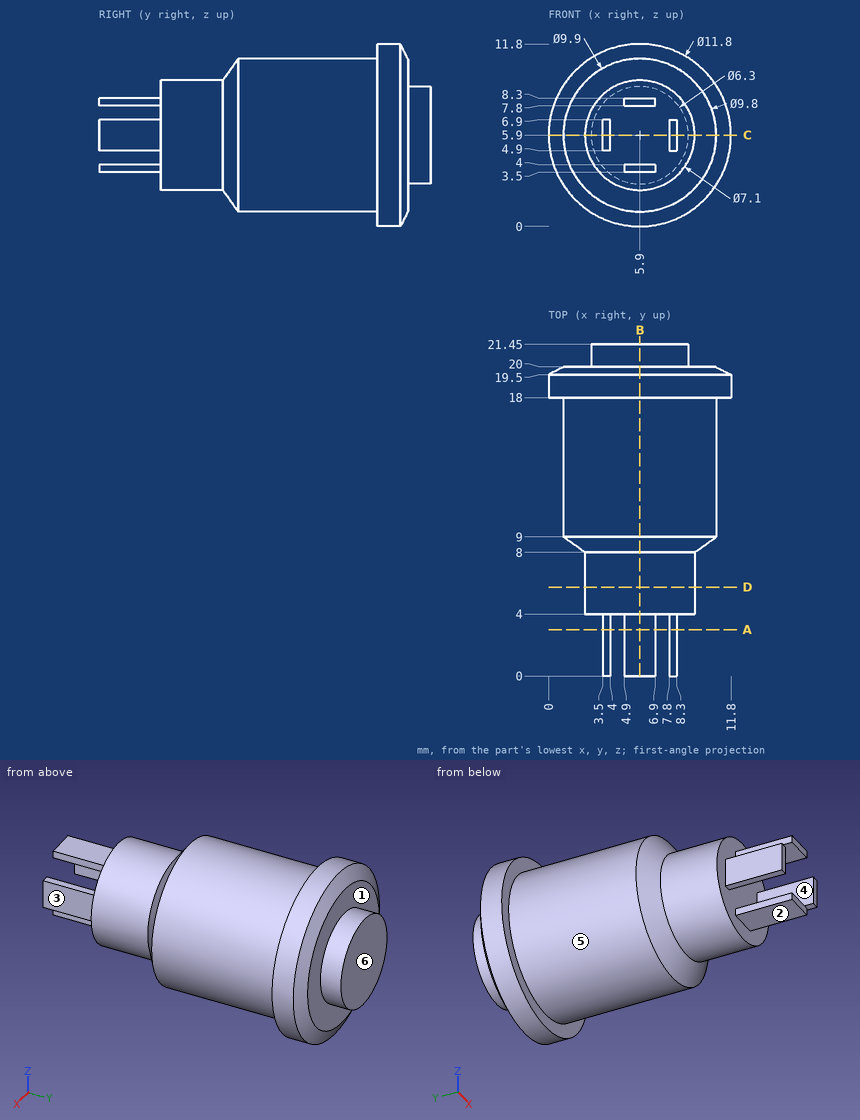
Input: dimensioned drawing with shaded views. Units: mm. Origin: part minimum x, y, z. A direction names the side the tool comes from. Coordinates: 2 decimals unless noted, no trailing zeros. Write each loop counter-clockwise with the first axis right and the second up, starting at its lowest first coordinate (ties: lowest second). Pieces come first, ordered by that corner, then holes. Notation, with made-up numbers: M 74.5,48.25 L 88.5,48.25 A34 cw 88.5,78.25 Z; hole C -12,-29.75 d1. An arc over 180 degrees is marked long. Answer as CSV lines item,"result". Start each with the question number.
Q1. Cut plane D-D on y = 5.75. Return the cut outline in (x, z), then the cut area to 3 significant figures.
Q2. Line query: line 1 (Y direction, x = 4.75, z = 7.5); line 2 (X direction, y = 2.5, z = 8); line 3 (X direction, y = 13.5, z = 4.75). Output: solid intervals per line, ascending. Write a range as from..to.
Q3. Cut plane A-A on y = 3. Return the cut outline in (x, z), then the cut area to 3 significant figures.
Q4. Cut plane C-C on z = 5.9. Return the cut outline in (x, y), then the cut area to 3 significant figures.
Q5. Pin query (flat end, axial travel): P1, Ø6, axis at y = 12.5, z = 1.5, coming from the -X side; P2, Ø0.6, axis at x = 8, y = 1, coming from the -Z side; P3, Ø2, axis at x = 6, y = 2.5, coming from the +Z side. Return the tip coordinate at first contact, or that it passes through.
Q6. Cut plane B-B on x = 5.9. Return the cut outline in (y, z).
Q7. Reachability of the marked faces 1, 2 and 3 from +Z, -Z, +X, -X, +Y, -Y: full face, straight path, thin tool, end or side. Return the list, or none.
Q8. Mould query, pull axis X, two halves, no side actions, for the marked faces 4, 5 and 6. Classes: released by +X, released by -X, zero draft, split by the parting line, or undercut.
Findings below:
1,outline,"C 5.9,5.9 d7.1"
1,area,"39.6 mm2"
2,line 1,"y = 4..21.45"
2,line 2,"x = 4.9..6.9"
2,line 3,"x = 1.09..10.71"
3,outline,"M 3.5,4.9 L 4,4.9 L 4,6.9 L 3.5,6.9 Z; M 4.9,3.5 L 6.9,3.5 L 6.9,4 L 4.9,4 Z; M 4.9,7.8 L 6.9,7.8 L 6.9,8.3 L 4.9,8.3 Z; M 7.8,4.9 L 8.3,4.9 L 8.3,6.9 L 7.8,6.9 Z"
3,area,"4.00 mm2"
4,outline,"M 0,18 L 0.95,18 L 0.95,9 L 2.35,8 L 2.35,4 L 3.5,4 L 3.5,0 L 4,0 L 4,4 L 7.8,4 L 7.8,0 L 8.3,0 L 8.3,4 L 9.45,4 L 9.45,8 L 10.85,9 L 10.85,18 L 11.8,18 L 11.8,19.5 L 10.8,20 L 9.05,20 L 9.05,21.45 L 2.75,21.45 L 2.75,20 L 1,20 L 0,19.5 Z"
4,area,"162 mm2"
5,P1,"stops at x = 1.15"
5,P2,"stops at z = 4.9"
5,P3,"stops at z = 8.3"
6,outline,"M 0,3.5 L 4,3.5 L 4,2.35 L 8,2.35 L 9,0.95 L 18,0.95 L 18,0 L 19.5,0 L 20,1 L 20,2.75 L 21.45,2.75 L 21.45,9.05 L 20,9.05 L 20,10.8 L 19.5,11.8 L 18,11.8 L 18,10.85 L 9,10.85 L 8,9.45 L 4,9.45 L 4,8.3 L 0,8.3 L 0,7.8 L 4,7.8 L 4,4 L 0,4 Z"
7,face 1,"+Y"
7,face 2,"-Z, +X, -X, -Y"
7,face 3,"+Z, -Z, +X, -Y"
8,face 4,"undercut"
8,face 5,"split by the parting line"
8,face 6,"zero draft"
